Geometry: final body of the model. Coordinates: model frame, mm. Coordinates: 2 decimals unless noted, no trailing zeros. Order: outer loops, then holes, each group sorted by start corner. A loop starts at its lowest first (then second) coordinate and runs counter-clockwise, first axis right, second up. Notation, with made-up numbers: (4, 4.5) -> (11, 4.5) arc R22 ccw to (11, 25.5) -> close; hole circle Ø1 at (75, 11). An arc over 180 degrees is marked (long way). Use one line per item in the form item = value.
```python
from build123d import *

# Parameters (mm, degrees)
SKETCH_1_W      = 10
SKETCH_1_H      = 5
SKETCH_1_W_2    = 20
SKETCH_1_W_3    = 5
SKETCH_1_H_2    = 10
EXTRUDE_1_DEPTH = 5


with BuildPart() as part:
    # 草图1 → 凸台-拉伸1 (new body)
    with BuildSketch(Plane(origin=(0, 0, 0), x_dir=(1, 0, 0), z_dir=(0, 1, 0))):
        Polygon((-195.058737628, 90.053763441), (76.941262372, 90.053763441), (81.941262372, 90.053763441), (81.941262372, -43.946236559), (76.941262372, -43.946236559), (-195.058737628, -43.946236559), align=None)
        with Locations((61.941262372, 37.553763441)):
            Rectangle(SKETCH_1_W, SKETCH_1_H, mode=Mode.SUBTRACT)
        with Locations((-142.058737628, 37.553763441)):
            Rectangle(SKETCH_1_W, SKETCH_1_H, mode=Mode.SUBTRACT)
        with Locations((-142.058737628, -36.446236559)):
            Rectangle(SKETCH_1_W, SKETCH_1_H, mode=Mode.SUBTRACT)
        with Locations((61.941262372, -36.446236559)):
            Rectangle(SKETCH_1_W, SKETCH_1_H, mode=Mode.SUBTRACT)
        with Locations((-40.058737628, 37.553763441)):
            Rectangle(SKETCH_1_W_2, SKETCH_1_H, mode=Mode.SUBTRACT)
        with Locations((-154.558737628, 20.053763441)):
            Rectangle(SKETCH_1_W_3, SKETCH_1_H_2, mode=Mode.SUBTRACT)
        with Locations((-154.558737628, -18.946236559)):
            Rectangle(SKETCH_1_W_3, SKETCH_1_H_2, mode=Mode.SUBTRACT)
        with Locations((74.441262372, 20.053763441)):
            Rectangle(SKETCH_1_W_3, SKETCH_1_H_2, mode=Mode.SUBTRACT)
        with Locations((74.441262372, -18.946236559)):
            Rectangle(SKETCH_1_W_3, SKETCH_1_H_2, mode=Mode.SUBTRACT)
        with Locations((-40.058737628, -36.446236559)):
            Rectangle(SKETCH_1_W_2, SKETCH_1_H, mode=Mode.SUBTRACT)
        with Locations((-120.558737628, 20.053763441)):
            Rectangle(SKETCH_1_W_3, SKETCH_1_H_2, mode=Mode.SUBTRACT)
        with Locations((-120.558737628, -18.946236559)):
            Rectangle(SKETCH_1_W_3, SKETCH_1_H_2, mode=Mode.SUBTRACT)
    extrude(amount=EXTRUDE_1_DEPTH)


solid = part.part
```
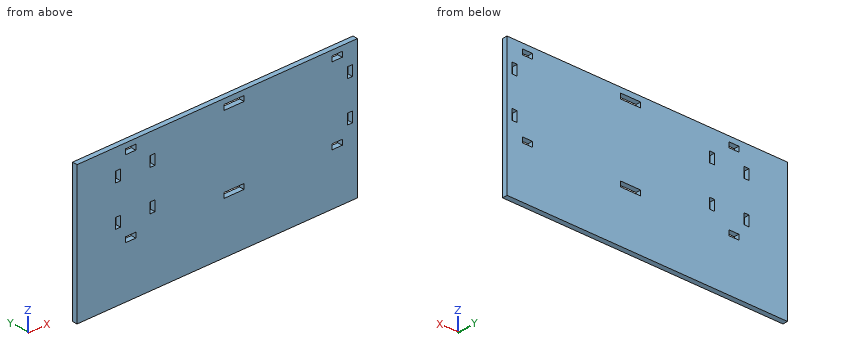
1) Section A-A, the plane x = -43. Output: boundary loops of the cut face in (y, z), and give its area (3 significant figures).
Results found:
outline = (0, -90.05) -> (5, -90.05) -> (5, -40.05) -> (0, -40.05) -> close; (0, -35.05) -> (5, -35.05) -> (5, 33.95) -> (0, 33.95) -> close; (0, 38.95) -> (5, 38.95) -> (5, 43.95) -> (0, 43.95) -> close
area = 620 mm2
2) Material intervals for probe 1 along X at (y, z) = (1.45, -25); probe 2 along Z at (x, y) = (62.5, 1.3); probe 3 along Z at (x, y) = (-155, 0.75), sorted ascending. Write a range as from..to.
Results found:
probe_1 = -195.06..-157.06, -152.06..-123.06, -118.06..71.94, 76.94..81.94
probe_2 = -90.05..-40.05, -35.05..33.95, 38.95..43.95
probe_3 = -90.05..-25.05, -15.05..13.95, 23.95..43.95
3) Section B-B, the plane y = 1.85. Give the number of separate pieces and of enclosed holes in the cut face, and give its area (3 significant figures).
Results found:
separate_pieces = 1
enclosed_holes = 12
area = 36,400 mm2
